```python
from build123d import *

# Parameters (mm, degrees)
SKETCH1_W           = 45
SKETCH1_H           = 30
BOSS_EXTRUDE1_DEPTH = 25
SKETCH2_R           = 9
BOSS_EXTRUDE2_DEPTH = 30


with BuildPart() as part:
    # Sketch1 → Boss-Extrude1 (new body)
    with BuildSketch(Plane.XY):
        Rectangle(SKETCH1_W, SKETCH1_H)
    extrude(amount=BOSS_EXTRUDE1_DEPTH)

    # Sketch2 → Boss-Extrude2 (add)
    with BuildSketch(Plane(origin=(0, 15, 0), x_dir=(1, 0, 0), z_dir=(0, 1, 0))):
        with Locations((13.5, -12.5)):
            Circle(SKETCH2_R)
    extrude(amount=BOSS_EXTRUDE2_DEPTH)


solid = part.part
```
Model file for the job. Use its own axes, mm. A direction names the side the tool comes from. Round coordinates to 2 decimals unless told otherwise and drop trailing zeros. Order: outer loops, then holes, each group sorted by start corner. A loop starts at its lowest first (then second) coordinate and runs counter-clockwise, first axis right, second up. Notation, with made-up numbers: (1.25, 79) -> (34.25, 79) arc R21 ccw to (34.25, 97) -> close; hole circle Ø9 at (46.5, -15.5). An arc over 180 degrees is marked (long way). Use one line per item in the form item = value.
Item 1: Cut at B-B, the plane z = 11. Write the cut outline in (x, y).
Returned:
outline = (-22.5, -15) -> (22.5, -15) -> (22.5, 15) -> (22.37, 15) -> (22.37, 45) -> (4.63, 45) -> (4.63, 15) -> (-22.5, 15) -> close
Item 2: Drill centre lines: line 1 (Y direction, x = 0, z = 15.25); line 2 (X direction, y = 27, z = 13); line 3 (Z direction, x = 9, y = 22). Where is each one in solid material? Low to high.
Returned:
line_1 = -15 to 15
line_2 = 4.51 to 22.49
line_3 = 4.71 to 20.29
Item 3: Cut at C-C, the plane y = 31. Write the cut outline in (x, z).
Returned:
outline = circle Ø18 at (13.5, 12.5)
Item 4: Cut at D-D, the plane z = 2.75. Write the cut outline in (x, y), and give its area (3 significant figures).
Returned:
outline = (-22.5, -15) -> (22.5, -15) -> (22.5, 15) -> (-22.5, 15) -> close
area = 1,350 mm^2
Item 5: Cut at A-A, the plane x = 13.5. Write the cut outline in (y, z), and give its area (3 significant figures).
Returned:
outline = (-15, 0) -> (15, 0) -> (15, 3.5) -> (45, 3.5) -> (45, 21.5) -> (15, 21.5) -> (15, 25) -> (-15, 25) -> close
area = 1,290 mm^2
Item 6: Tool access for faces 1 (the face through (11.549, 29.79, 21.286)), 2 (the face through (22.5, 0, 12)): list every direction of +Z, -Z, +X, -X, +Y, -Y with a clear straight run to the whole face (end or side of a thin tool).
Returned:
face_1 = +Y
face_2 = +Z, -Z, +X, +Y, -Y
